from build123d import *

# Parameters (mm, degrees)
BOSS_EXTRUDE1_DEPTH = 2.7
CAVITY1_OUTLINE_W   = 30
CAVITY1_OUTLINE_H   = 2.7
CAVITY1_DEPTH       = 2.7
CAVITY2_START       = -11.622776602
CAVITY2_OUTLINE_W   = 1.798654648
CAVITY2_OUTLINE_H   = 2.7
CAVITY2_DEPTH       = 30
CAVITY2_START_2     = 108.377223398
CAVITY2_2_OUTLINE_W = 1.798654648
CAVITY2_2_OUTLINE_H = 2.7
CAVITY2_2_DEPTH     = 30
CAVITY2_START_3     = 228.377223398
CAVITY2_3_OUTLINE_W = 1.798654648
CAVITY2_3_OUTLINE_H = 2.7
CAVITY2_3_DEPTH     = 30
CUT_EXTRUDE1_DEPTH  = 317.239292309
BOSS_EXTRUDE3_DEPTH = 2.7
SKETCH7_R           = 0.25
CUT_EXTRUDE2_DEPTH  = 2.7
FILLET2_R           = 0.5


# Read off the part's stored shape, not the designer's step: Cavity1, Cavity2
with BuildPart() as part:
    # Sketch1 → Boss-Extrude1 (new body)
    with BuildSketch(Plane.XY):
        Polygon((0, 0), (300, 0), (0, 100), align=None)
    extrude(amount=BOSS_EXTRUDE1_DEPTH)

    # Cavity1 outline → Cavity1 (cut)
    with BuildSketch(Plane.XY):
        with Locations((30.21166892, 1.35)):
            Rectangle(CAVITY1_OUTLINE_W, CAVITY1_OUTLINE_H)
        Polygon((47.149134475, 83.333520418), (47.434164903, 84.188611699), (18.973665961, 93.67544468), (18.688635534, 92.820353398), align=None)
        Polygon((160.991130241, 45.386188495), (161.276160669, 46.241279777), (132.815661727, 55.728112758), (132.5306313, 54.873021476), align=None)
        Polygon((274.833126007, 7.438856573), (275.118156435, 8.293947855), (246.657657493, 17.780780836), (246.372627066, 16.925689554), align=None)
        with Locations((250.21166892, 1.35)):
            Rectangle(CAVITY1_OUTLINE_W, CAVITY1_OUTLINE_H)
        with Locations((140.21166892, 1.35)):
            Rectangle(CAVITY1_OUTLINE_W, CAVITY1_OUTLINE_H)
    extrude(amount=CAVITY1_DEPTH, mode=Mode.SUBTRACT)

    # Cavity2 outline → Cavity2 (cut)
    with BuildSketch(Plane(origin=(0, 0, 0), x_dir=(0.316227766016832, 0.9486832980505158, 0), z_dir=(0.9486832980505159, -0.316227766016832, 0)).offset(CAVITY2_START)):
        with Locations((93.067657129, 1.35)):
            Rectangle(CAVITY2_OUTLINE_W, CAVITY2_OUTLINE_H)
    extrude(amount=CAVITY2_DEPTH, mode=Mode.SUBTRACT)

    # Cavity2 2 outline → Cavity2 2 (cut)
    with BuildSketch(Plane(origin=(0, 0, 0), x_dir=(0.316227766016832, 0.9486832980505158, 0), z_dir=(0.9486832980505159, -0.316227766016832, 0)).offset(CAVITY2_START_2)):
        with Locations((93.067657129, 1.35)):
            Rectangle(CAVITY2_2_OUTLINE_W, CAVITY2_2_OUTLINE_H)
    extrude(amount=CAVITY2_2_DEPTH, mode=Mode.SUBTRACT)

    # Cavity2 3 outline → Cavity2 3 (cut)
    with BuildSketch(Plane(origin=(0, 0, 0), x_dir=(0.316227766016832, 0.9486832980505158, 0), z_dir=(0.9486832980505159, -0.316227766016832, 0)).offset(CAVITY2_START_3)):
        with Locations((93.067657129, 1.35)):
            Rectangle(CAVITY2_3_OUTLINE_W, CAVITY2_3_OUTLINE_H)
    extrude(amount=CAVITY2_3_DEPTH, mode=Mode.SUBTRACT)

    # Sketch4 → Cut-Extrude1 (cut, through all)
    with BuildSketch(Plane.XY.offset(2.7)):
        Polygon((292.315665286, 2.561444905), (291.461850318, 0), (300, 0), align=None)
    extrude(amount=-CUT_EXTRUDE1_DEPTH, mode=Mode.SUBTRACT)

    # Sketch5 → Boss-Extrude3 (add)
    with BuildSketch(Plane.XY.offset(2.7)):
        Polygon((0, 100), (-0.853814968, 97.438555095), (-0.426907484, 0), (0, 0), align=None)
    extrude(amount=-BOSS_EXTRUDE3_DEPTH)

    # Sketch7 → Cut-Extrude2 (cut)
    with BuildSketch(Plane.XY.offset(2.7)):
        with Locations((18.343457791, 91.225803174)):
            Circle(SKETCH7_R)
        with Locations((132.185453557, 53.278471252)):
            Circle(SKETCH7_R)
        with Locations((46.468546535, 81.850773592)):
            Circle(SKETCH7_R)
        with Locations((160.310542301, 43.90344167)):
            Circle(SKETCH7_R)
        with Locations((246.027449323, 15.33113933)):
            Circle(SKETCH7_R)
        with Locations((274.152538068, 5.956109748)):
            Circle(SKETCH7_R)
        with Locations((265.034892224, 2.523223305)):
            Circle(SKETCH7_R)
        with Locations((235.388445615, 2.523223305)):
            Circle(SKETCH7_R)
        with Locations((155.034892224, 2.523223305)):
            Circle(SKETCH7_R)
        with Locations((125.388445615, 2.523223305)):
            Circle(SKETCH7_R)
        with Locations((45.034892224, 2.523223305)):
            Circle(SKETCH7_R)
        with Locations((15.388445615, 2.523223305)):
            Circle(SKETCH7_R)
    extrude(amount=-CUT_EXTRUDE2_DEPTH, mode=Mode.SUBTRACT)

    # Fillet2
    fillet2_edges = [part.edges().sort_by_distance(p)[0] for p in [
        (18.973665961, 93.67544468, 1.35),
        (47.434164903, 84.188611699, 1.35),
        (132.815661727, 55.728112758, 1.35),
        (161.276160669, 46.241279777, 1.35),
        (246.657657493, 17.780780836, 1.35),
        (275.118156435, 8.293947855, 1.35),
        (235.21166892, 0, 1.35),
        (125.21166892, 0, 1.35),
        (15.21166892, 0, 1.35),
        (265.21166892, 0, 1.35),
        (155.21166892, 0, 1.35),
        (45.21166892, 0, 1.35),
    ]]
    fillet(fillet2_edges, radius=FILLET2_R)


solid = part.part
Can you work these out from the model? Positions are in its coordinate system, mm. Coordinates: 2 decimals unless noted, no trailing zeros. Loops run counter-clockwise (first coordinate to the right, second up) from the corner with the lowest first, then second, coordinate; pieces in that order, holes last. Notation, with made-up numbers: M -30.75,59 L 16.25,59 A22 cw 16.25,82 Z; hole C -8.75,81.25 d3. An arc over 180 degrees is marked long. Answer as CSV lines item,"result". Start each with the question number.
1. Suppose I cut it at A-A, the plane x = 180. List the corners of the cut face in (y, z) for me, plus the area to 3 significant figures.
2. If I drill on probe 1 along Y at (x, z) = (210, 0.55); probe 2 along Y at (x, z) = (53.5, 2.2), over which ranges is the centre line in solid material (lowest first)? Write a range as [from, to].
3. Suppose I cut it at B-B, the plane y = 49.5. List the corners of the cut face in (x, z) for me, plus the area to 3 significant figures.
4. For pin 1 Ø1.5 at (x, z) = (30.5, 0.5) entering from +Y; pin 2 Ø0.6 at (y, z) = (1, 1) entering from -X; pin 3 Ø0.8 at (x, z) = (145.5, 1.5) entering from -Y, each with a flat end and sliding along its axis, tell me the tip position at first contact or that it passes through.
Output:
1,outline,"M 0,0 L 40,0 L 40,2.7 L 0,2.7 Z"
1,area,"108 mm^2"
2,probe 1,"y = [0, 30]"
2,probe 2,"y = [0, 82.17]"
3,outline,"M -0.64,0 L 142.96,0 L 142.96,2.7 L -0.64,2.7 Z"
3,area,"388 mm^2"
4,pin 1,"stops at y = 87.24"
4,pin 2,"stops at x = -0.43"
4,pin 3,"stops at y = 2.7"
